```python
from build123d import *

# Parameters (mm, degrees)
F1_DEPTH = 3.175
F2_R     = 3.175
F3_DEPTH = 25.4
F4_R     = 2.54
F5_DEPTH = 3.176


with BuildPart() as f1:
    # F0 (on Top) → F1 (new body)
    with BuildSketch(Plane.XY):
        Polygon((29.745836, 88.9), (-29.745836, 88.9), (-63.5, 48.554318), (-63.5, -48.554318), (-29.745836, -88.9), (29.745836, -88.9), (63.5, -48.554318), (63.5, 48.554318), align=None)
    extrude(amount=F1_DEPTH)

    # F2 (on face) → F3 (cut)
    with BuildSketch(Plane.XY.offset(3.175)):
        with Locations((-43.392069, 57.744911)):
            Circle(F2_R)
        with Locations((-35.242826, 67.48554)):
            Circle(F2_R)
        with Locations((35.242824, 67.485542)):
            Circle(F2_R)
        with Locations((43.392067, 57.744913)):
            Circle(F2_R)
        with Locations((43.392069, -57.744911)):
            Circle(F2_R)
        with Locations((35.242826, -67.48554)):
            Circle(F2_R)
        with Locations((-35.242826, -67.48554)):
            Circle(F2_R)
        with Locations((-43.392069, -57.744911)):
            Circle(F2_R)
    extrude(amount=-F3_DEPTH, mode=Mode.SUBTRACT)

    # F4 (on face) → F5 (cut, through all)
    with BuildSketch(Plane.XY.offset(3.175)):
        with Locations((-22.225, 22.225)):
            Circle(F4_R)
        with Locations((22.225, 22.225)):
            Circle(F4_R)
        with Locations((-22.225, -22.225)):
            Circle(F4_R)
        with Locations((22.225, -22.225)):
            Circle(F4_R)
    extrude(amount=-F5_DEPTH, mode=Mode.SUBTRACT)


solid = f1.part
```
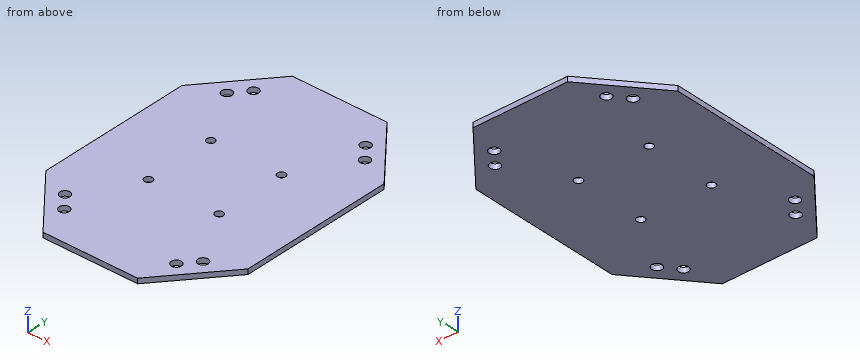
Verification items for the finished model (mm, model axes). Give positions to 0.01 mm unless a question says otherwise; leave off trailing zeros. Loops run counter-clockwise (first coordinate to the right, second up) from the corner with the lowest first, then second, coordinate; pieces in that order, holes last. Notation, with made-up numbers: M 85.25,5.5 L 137.25,5.5 A21 cw 137.25,27.5 Z; hole C 59.5,48.25 d4. An arc over 180 degrees is marked long. Return JSON: item names as keys, results as strings.
1) Section check C-C, the plane x = 23. Enter the section's corners in (y, z) (3 decimals).
Findings:
{"outline": "M -88.9,0 L -24.644,0 L -24.644,3.175 L -88.9,3.175 Z; M -19.806,0 L 19.806,0 L 19.806,3.175 L -19.806,3.175 Z; M 24.644,0 L 88.9,0 L 88.9,3.175 L 24.644,3.175 Z"}
2) Section check D-D, the plane x = 52.5. Enter the section's corners in (y, z) (3 decimals).
Findings:
{"outline": "M -61.702,0 L 61.702,0 L 61.702,3.175 L -61.702,3.175 Z"}
3) Gauge pin test, flat end, axial feed: P1, Ø5.5, axis at x = -43.39, y = 57.74, coming from the -Z side. Record the tip position at first contact, or that the pin passes through.
Findings:
{"P1": "passes through"}
4) Section check B-B, the plane z = 2.5. Count the separate pieces of the cut face and the enclosed holes in it, and give its area (3 significant figures).
Findings:
{"separate pieces": "1", "enclosed holes": "12", "area": "19,500 mm2"}
5) Section check A-A, the plane x = 36. Enter the section's corners in (y, z) (3 decimals), and give its area (3 significant figures).
Findings:
{"outline": "M -81.425,0 L -70.569,0 L -70.569,3.175 L -81.425,3.175 Z; M -64.402,0 L 64.402,0 L 64.402,3.175 L -64.402,3.175 Z; M 70.569,0 L 81.425,0 L 81.425,3.175 L 70.569,3.175 Z", "area": "478 mm2"}
6) Material ranges on L1, parallel to Y at x = -24, z = 2.1; L2, parallel to Y at x = -23.5, z = 2.2; L3, parallel to X at y = -59.5, z = 0.9, recorded low to high. Write a range as [from, to].
Findings:
{"L1": "y = [-88.9, -24.04], [-20.41, 20.41], [24.04, 88.9]", "L2": "y = [-88.9, -24.42], [-20.03, 20.03], [24.42, 88.9]", "L3": "x = [-54.34, -46.04], [-40.75, 40.75], [46.04, 54.34]"}
